```python
from build123d import *

# Parameters (mm, degrees)
BOX003_W        = 20
BOX003_H        = 10
BOX003_DEPTH    = 2
CHAMFER003_SIZE = 1.9
BOX004_W        = 20
BOX004_H        = 10
BOX004_DEPTH    = 2
CHAMFER004_SIZE = 1.9
BOX005_W        = 20
BOX005_H        = 10
BOX005_DEPTH    = 2
CHAMFER005_SIZE = 1.9
BOX006_W        = 20
BOX006_H        = 10
BOX006_DEPTH    = 2
CHAMFER006_SIZE = 1.9
BOX007_W        = 20
BOX007_H        = 10
BOX007_DEPTH    = 2
CHAMFER007_SIZE = 1.9
BOX008_W        = 20
BOX008_H        = 10
BOX008_DEPTH    = 2
CHAMFER008_SIZE = 1.9
BOX009_W        = 64
BOX009_H        = 34
BOX009_DEPTH    = 2
BOX002_W        = 20
BOX002_H        = 10
BOX002_DEPTH    = 2
CHAMFER002_SIZE = 1.9
BOX001_W        = 20
BOX001_H        = 10
BOX001_DEPTH    = 2
CHAMFER001_SIZE = 1.9
BOX_W           = 20
BOX_H           = 10
BOX_DEPTH       = 2
CHAMFER_SIZE    = 1.9


with BuildPart() as chamfer003:
    # Box003 → Box003 (new body)
    with BuildSketch(Plane.XY):
        with Locations((10, 5)):
            Rectangle(BOX003_W, BOX003_H)
    extrude(amount=BOX003_DEPTH)

    # Chamfer003
    chamfer003_edges = [chamfer003.edges().sort_by_distance(p)[0] for p in [
        (0, 5, 2),
        (20, 5, 2),
        (10, 0, 2),
        (10, 10, 2),
    ]]
    chamfer(chamfer003_edges, length=CHAMFER003_SIZE)


with BuildPart() as chamfer003_1:
    # Chamfer003 placement: moved
    add(chamfer003.part.moved(Location((0, 12, 0))))


with BuildPart() as chamfer004:
    # Box004 → Box004 (new body)
    with BuildSketch(Plane.XY):
        with Locations((10, 5)):
            Rectangle(BOX004_W, BOX004_H)
    extrude(amount=BOX004_DEPTH)

    # Chamfer004
    chamfer004_edges = [chamfer004.edges().sort_by_distance(p)[0] for p in [
        (0, 5, 2),
        (20, 5, 2),
        (10, 0, 2),
        (10, 10, 2),
    ]]
    chamfer(chamfer004_edges, length=CHAMFER004_SIZE)


with BuildPart() as chamfer004_1:
    # Chamfer004 placement: moved
    add(chamfer004.part.moved(Location((22, 12, 0))))


with BuildPart() as chamfer005:
    # Box005 → Box005 (new body)
    with BuildSketch(Plane.XY):
        with Locations((10, 5)):
            Rectangle(BOX005_W, BOX005_H)
    extrude(amount=BOX005_DEPTH)

    # Chamfer005
    chamfer005_edges = [chamfer005.edges().sort_by_distance(p)[0] for p in [
        (0, 5, 2),
        (20, 5, 2),
        (10, 0, 2),
        (10, 10, 2),
    ]]
    chamfer(chamfer005_edges, length=CHAMFER005_SIZE)


with BuildPart() as chamfer005_1:
    # Chamfer005 placement: moved
    add(chamfer005.part.moved(Location((44, 12, 0))))


with BuildPart() as chamfer006:
    # Box006 → Box006 (new body)
    with BuildSketch(Plane.XY):
        with Locations((10, 5)):
            Rectangle(BOX006_W, BOX006_H)
    extrude(amount=BOX006_DEPTH)

    # Chamfer006
    chamfer006_edges = [chamfer006.edges().sort_by_distance(p)[0] for p in [
        (0, 5, 2),
        (20, 5, 2),
        (10, 0, 2),
        (10, 10, 2),
    ]]
    chamfer(chamfer006_edges, length=CHAMFER006_SIZE)


with BuildPart() as chamfer006_1:
    # Chamfer006 placement: moved
    add(chamfer006.part.moved(Location((0, 24, 0))))


with BuildPart() as chamfer007:
    # Box007 → Box007 (new body)
    with BuildSketch(Plane.XY):
        with Locations((10, 5)):
            Rectangle(BOX007_W, BOX007_H)
    extrude(amount=BOX007_DEPTH)

    # Chamfer007
    chamfer007_edges = [chamfer007.edges().sort_by_distance(p)[0] for p in [
        (0, 5, 2),
        (20, 5, 2),
        (10, 0, 2),
        (10, 10, 2),
    ]]
    chamfer(chamfer007_edges, length=CHAMFER007_SIZE)


with BuildPart() as chamfer007_1:
    # Chamfer007 placement: moved
    add(chamfer007.part.moved(Location((22, 24, 0))))


with BuildPart() as chamfer008:
    # Box008 → Box008 (new body)
    with BuildSketch(Plane.XY):
        with Locations((10, 5)):
            Rectangle(BOX008_W, BOX008_H)
    extrude(amount=BOX008_DEPTH)

    # Chamfer008
    chamfer008_edges = [chamfer008.edges().sort_by_distance(p)[0] for p in [
        (0, 5, 2),
        (20, 5, 2),
        (10, 0, 2),
        (10, 10, 2),
    ]]
    chamfer(chamfer008_edges, length=CHAMFER008_SIZE)


with BuildPart() as chamfer008_1:
    # Chamfer008 placement: moved
    add(chamfer008.part.moved(Location((44, 24, 0))))


with BuildPart() as cubo009:
    # Box009 → Box009 (new body)
    with BuildSketch(Plane.XY.offset(-2)):
        with Locations((32, 17)):
            Rectangle(BOX009_W, BOX009_H)
    extrude(amount=BOX009_DEPTH)


with BuildPart() as chamfer002:
    # Box002 → Box002 (new body)
    with BuildSketch(Plane.XY):
        with Locations((10, 5)):
            Rectangle(BOX002_W, BOX002_H)
    extrude(amount=BOX002_DEPTH)

    # Chamfer002
    chamfer002_edges = [chamfer002.edges().sort_by_distance(p)[0] for p in [
        (0, 5, 2),
        (20, 5, 2),
        (10, 0, 2),
        (10, 10, 2),
    ]]
    chamfer(chamfer002_edges, length=CHAMFER002_SIZE)


with BuildPart() as chamfer002_1:
    # Chamfer002 placement: moved
    add(chamfer002.part.moved(Location((44, 0, 0))))


with BuildPart() as chamfer001:
    # Box001 → Box001 (new body)
    with BuildSketch(Plane.XY):
        with Locations((10, 5)):
            Rectangle(BOX001_W, BOX001_H)
    extrude(amount=BOX001_DEPTH)

    # Chamfer001
    chamfer001_edges = [chamfer001.edges().sort_by_distance(p)[0] for p in [
        (0, 5, 2),
        (20, 5, 2),
        (10, 0, 2),
        (10, 10, 2),
    ]]
    chamfer(chamfer001_edges, length=CHAMFER001_SIZE)


with BuildPart() as chamfer001_1:
    # Chamfer001 placement: moved
    add(chamfer001.part.moved(Location((22, 0, 0))))


with BuildPart() as fusion:
    # Box → Box (new body)
    with BuildSketch(Plane.XY):
        with Locations((10, 5)):
            Rectangle(BOX_W, BOX_H)
    extrude(amount=BOX_DEPTH)

    # Chamfer
    chamfer_edges = [fusion.edges().sort_by_distance(p)[0] for p in [
        (0, 5, 2),
        (20, 5, 2),
        (10, 0, 2),
        (10, 10, 2),
    ]]
    chamfer(chamfer_edges, length=CHAMFER_SIZE)

    # Fusion: union Chamfer003, Chamfer004, Chamfer005, Chamfer006, Chamfer007, Chamfer008, Cubo009, Chamfer002, Chamfer001
    add(chamfer003_1.part)
    add(chamfer004_1.part)
    add(chamfer005_1.part)
    add(chamfer006_1.part)
    add(chamfer007_1.part)
    add(chamfer008_1.part)
    add(cubo009.part)
    add(chamfer002_1.part)
    add(chamfer001_1.part)


solid = fusion.part
```
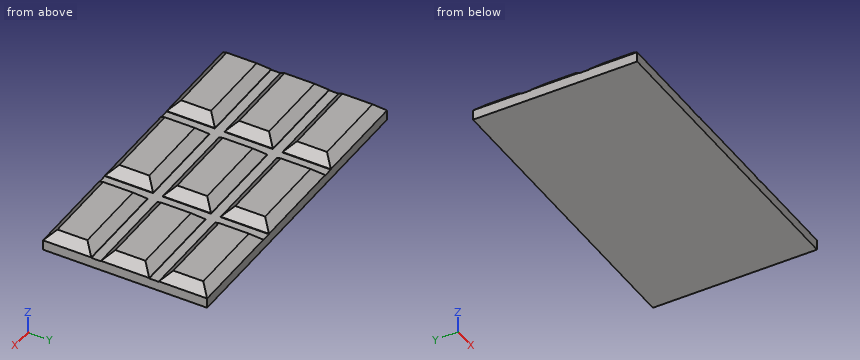
CAD build for the part. Positions are in the model's coordinates, mm. Round coordinates to 2 decimals unless told otherwise and drop trailing zeros. Order: outer loops, then holes, each group sorted by start corner. A loop starts at its lowest first (then second) coordinate and runs counter-clockwise, first axis right, second up. Notation, with made-up numbers: (-2.75, 36.25) - (43.25, 36.25) arc R5 cw to (43.25, 42.25) - close; hole circle Ø3 at (-9.75, -7). An arc over 180 degrees is marked (long way). Answer as CSV lines item,"result". Start each with the question number.
1. Pin check, flat tips, straight feed: pin 1 (1 mm diameter, centred on x = 9.5, y = 21.5, fed in from +Z); pin 2 (1.5 mm diameter, centred on x = 51, z = -0.5, fed in from -Y). Stop position of each tip, or through.
2. Saw through at B-B, the plane y = 9. Write the cut outline in (x, z).
3. Drill centre lines: L1, parallel to X at y = 16.5, z = 0.1; L2, parallel to Y at x = 27.5, z = 0.8; L3, parallel to Y at x = 37, z = 1.85. Where is each one in solid material? Low to high. Write a range as [from, to].
4. Saw through at A-A, the plane x = 28.5. Write the cut outline in (y, z).
5. Saw through at C-C, the plane z = 1.1. Count the separate pieces of the cut face and the enclosed holes in it, and give its area (3 significant figures).
Model answer:
1,pin 1,"stops at z = 1.1"
1,pin 2,"stops at y = 0"
2,outline,"(0, -2) - (64, -2) - (64, 0.1) - (63, 1.1) - (45, 1.1) - (44, 0.1) - (44, 0) - (42, 0) - (42, 0.1) - (41, 1.1) - (23, 1.1) - (22, 0.1) - (22, 0) - (20, 0) - (20, 0.1) - (19, 1.1) - (1, 1.1) - (0, 0.1) - close"
3,L1,"x = [0, 20], [22, 42], [44, 64]"
3,L2,"y = [0.7, 9.3], [12.7, 21.3], [24.7, 33.3]"
3,L3,"y = [1.75, 8.25], [13.75, 20.25], [25.75, 32.25]"
4,outline,"(0, -2) - (34, -2) - (34, 0.1) - (32.1, 2) - (25.9, 2) - (24, 0.1) - (24, 0) - (22, 0) - (22, 0.1) - (20.1, 2) - (13.9, 2) - (12, 0.1) - (12, 0) - (10, 0) - (10, 0.1) - (8.1, 2) - (1.9, 2) - (0, 0.1) - close"
5,separate pieces,"9"
5,enclosed holes,"0"
5,area,"1,300 mm²"
